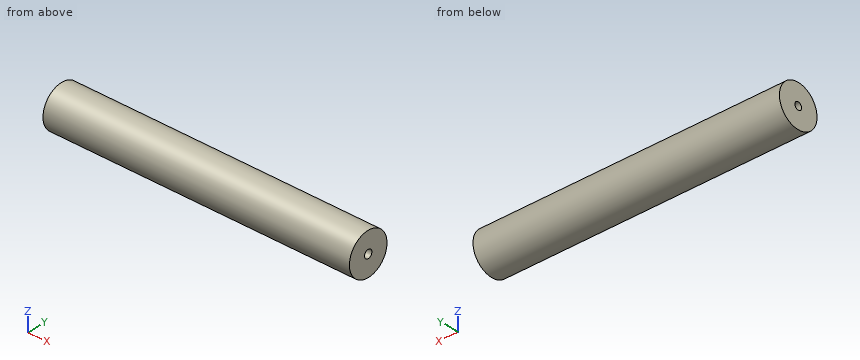
```python
from build123d import *

# Parameters (mm, degrees)
SKETCH1_R                       = 38.1
BOSS_EXTRUDE1_DEPTH             = 558.8
M12_CLEARANCE_HOLE1_D           = 13.5
M12_CLEARANCE_HOLE1_DEPTH       = 21.344190822
M12_CLEARANCE_HOLE1_CSINK_D     = 13.55
M12_CLEARANCE_HOLE1_CSINK_ANGLE = 90
M12_CLEARANCE_HOLE1_TIP         = 4.055809178
M12_CLEARANCE_HOLE2_D           = 15
M12_CLEARANCE_HOLE2_DEPTH       = 20.893545357
M12_CLEARANCE_HOLE2_TIP         = 4.506454643


with BuildPart() as part:
    # Sketch1 → Boss-Extrude1 (new body)
    with BuildSketch(Plane(origin=(0, 0, 0), x_dir=(0, 0, -1), z_dir=(1, 0, 0))):
        Circle(SKETCH1_R)
    extrude(amount=BOSS_EXTRUDE1_DEPTH)

    # M12 Clearance Hole1
    with Locations(Plane.ZY):
        with Locations((0, 0)):
            CounterSinkHole(M12_CLEARANCE_HOLE1_D / 2, M12_CLEARANCE_HOLE1_CSINK_D / 2, depth=M12_CLEARANCE_HOLE1_DEPTH, counter_sink_angle=M12_CLEARANCE_HOLE1_CSINK_ANGLE)
            with Locations((0, 0, -(M12_CLEARANCE_HOLE1_DEPTH + M12_CLEARANCE_HOLE1_TIP / 2))):  # 118° drill point
                Cone(0, M12_CLEARANCE_HOLE1_D / 2, M12_CLEARANCE_HOLE1_TIP, mode=Mode.SUBTRACT)

    # M12 Clearance Hole2
    with Locations(Plane(origin=(558.8, 0, 0), x_dir=(0, 0, -1), z_dir=(1, 0, 0))):
        with Locations((0, 0)):
            Hole(M12_CLEARANCE_HOLE2_D / 2, depth=M12_CLEARANCE_HOLE2_DEPTH)
            with Locations((0, 0, -(M12_CLEARANCE_HOLE2_DEPTH + M12_CLEARANCE_HOLE2_TIP / 2))):  # 118° drill point
                Cone(0, M12_CLEARANCE_HOLE2_D / 2, M12_CLEARANCE_HOLE2_TIP, mode=Mode.SUBTRACT)


solid = part.part
```
Geometry: final body of the model. Coordinates: model frame, mm. Give positions to 0.01 mm unless a question says otherwise; leave off trailing zeros. Loops run counter-clockwise (first coordinate to the right, second up) from the corner with the lowest first, then second, coordinate; pieces in that order, holes last. Notation, with made-up numbers: (23.25, -12.5) -> (54.25, -12.5) arc R20 cw to (54.25, 4.5) -> close; hole circle Ø10 at (-11.5, -15). An arc over 180 degrees is marked (long way). Use one line per item in the form item = value.
Item 1: Section query C-C on y = 31.5. Output: boundary loops of the cut face in (x, z), and give its area (3 significant figures).
A:
outline = (0, -21.43) -> (558.8, -21.43) -> (558.8, 21.43) -> (0, 21.43) -> close
area = 24,000 mm^2
Item 2: Line query: probe 1 along Y at (x, z) = (11.75, 0); probe 2 along Y at (x, z) = (542, 0); probe 3 along Y at (x, z) = (293, 0.5). Output: solid intervals per line, ascending.
A:
probe_1 = -38.1 to -6.75, 6.75 to 38.1
probe_2 = -38.1 to -7.5, 7.5 to 38.1
probe_3 = -38.1 to 38.1
Item 3: Section query B-B on z = 15. Output: boundary loops of the cut face in (x, y).
A:
outline = (0, -35.02) -> (558.8, -35.02) -> (558.8, 35.02) -> (0, 35.02) -> close
Item 4: Section query A-A on x = 166.5. Output: boundary loops of the cut face in (y, z).
A:
outline = circle Ø76.2 at (0, 0)
Item 5: Pin query (flat end, axial travel): P1, Ø1.5, axis at x = 126.5, y = 14, coming from the -Z side; P2, Ø12, axis at x = 92.5, z = 11.5, coming from the -Y side; P3, Ø10, axis at x = 124, y = 27, coming from the -Z side. Return the tip coordinate at first contact, or that it passes through.
A:
P1 = -35.72
P2 = -37.7
P3 = -31.11
